Part model, mm, in its own coordinate system. Coordinates: 2 decimals unless noted, no trailing zeros. Write each loop counter-clockwise with the first axis right and the second up, starting at its lowest first coordinate (ties: lowest second). Pieces come first, ordered by that corner, then holes. Notation, with made-up numbers: (88, -9.75) -> (144, -9.75) arc R24 ccw to (144, 12.25) -> close; hole circle Ø2 at (-25.75, 19.25). An arc over 180 degrees is marked (long way). One line per question, with ' | ' between items. Start each with the question number.
Item 1: Saw through at A-A (y = 35). List the corners of the cut face in (x, z), and give its area (3 significant figures).
Item 2: Saw through at B-B (x = 141). List the corners of the cut face in (y, z), and give its area (3 significant figures).
Item 3: Probe probe 1 along Y at (x, z) = (23, 3.3); probe 2 along X at (y, z) = (54, 3); probe 3 along Y at (x, z) = (101, 1.9). List the from-to ranges inside material, lowest first. Write a range as [from, to].
Item 4: Pin check, flat tips, straight feed: pin 1 (0.9 mm diameter, centred on y = 111.5, z = 2.5, fed in from +X); pin 2 (1.5 mm diameter, centred on y = 4.5, z = 2, fed in from +X). Stop position of each tip, or through.
Item 5: Saw through at C-C (z = 0.9). List the corners of the cut face in (x, y).
from build123d import *

# Parameters (mm, degrees)
F0_W     = 162
F0_H     = 115
F0_W_2   = 151.84
F0_H_2   = 109.92
F1_DEPTH = 4
F2_R     = 6
F3_SIZE  = 12.7
F4_W     = 15
F4_H     = 4
F5_DEPTH = 6
F6_W     = 15
F6_H     = 4
F7_DEPTH = 6
F8_R     = 3


with BuildPart() as f1:
    # F0 (on Top) → F1 (new body)
    with BuildSketch(Plane.XY):
        with Locations((81, 57.5)):
            Rectangle(F0_W, F0_H)
        with Locations((81, 57.5)):
            Rectangle(F0_W_2, F0_H_2, mode=Mode.SUBTRACT)
    extrude(amount=F1_DEPTH)

    # F2
    f2_edges = [f1.edges().sort_by_distance(p)[0] for p in [
        (0, 115, 2),
        (162, 115, 2),
        (162, 0, 2),
        (0, 0, 2),
    ]]
    fillet(f2_edges, radius=F2_R)

    # F3
    f3_edges = [f1.edges().sort_by_distance(p)[0] for p in [
        (5.08, 112.46, 2),
        (156.92, 2.54, 2),
        (156.92, 112.46, 2),
        (5.08, 2.54, 2),
    ]]
    chamfer(f3_edges, length=F3_SIZE)

    # F4 (on face) → F5 (join)
    with BuildSketch(Plane(origin=(0, 2.54, 0), x_dir=(-1, 0, 0), z_dir=(0, 1, 0))):
        with Locations((-61, 2)):
            Rectangle(F4_W, F4_H)
    extrude(amount=F5_DEPTH)

    # F6 (on face) → F7 (join)
    with BuildSketch(Plane.XZ.offset(-112.46)):
        with Locations((101, 2)):
            Rectangle(F6_W, F6_H)
    extrude(amount=F7_DEPTH)

    # F8
    f8_edges = [f1.edges().sort_by_distance(p)[0] for p in [
        (93.5, 106.46, 2),
        (108.5, 106.46, 2),
        (68.5, 8.54, 2),
        (53.5, 8.54, 2),
    ]]
    fillet(f8_edges, radius=F8_R)


solid = f1.part
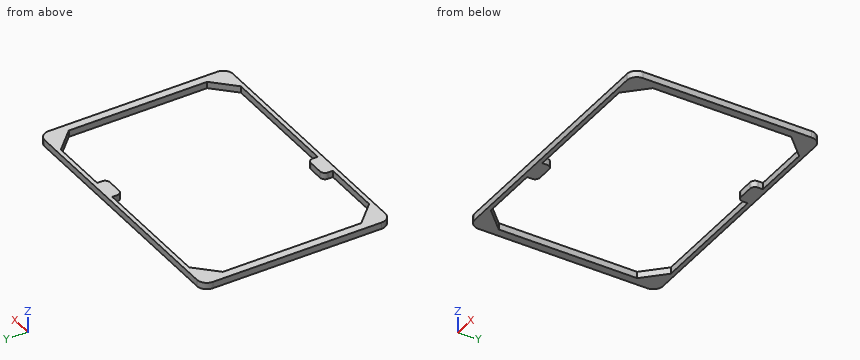
From the geometry:
1) outline: (0, 0) -> (5.08, 0) -> (5.08, 4) -> (0, 4) -> close; (156.92, 0) -> (162, 0) -> (162, 4) -> (156.92, 4) -> close | area: 40.6 mm2
2) outline: (0, 0) -> (2.54, 0) -> (2.54, 4) -> (0, 4) -> close; (112.46, 0) -> (115, 0) -> (115, 4) -> (112.46, 4) -> close | area: 20.3 mm2
3) probe 1: [0, 2.54], [112.46, 115] | probe 2: [0, 5.08], [156.92, 162] | probe 3: [0, 2.54], [106.46, 115]
4) pin 1: x = 161.64 | pin 2: x = 161.95
5) outline: (0, 6) arc R6 ccw to (6, 0) -> (156, 0) arc R6 ccw to (162, 6) -> (162, 109) arc R6 ccw to (156, 115) -> (6, 115) arc R6 ccw to (0, 109) -> close; hole (5.08, 15.24) -> (17.78, 2.54) -> (53.5, 2.54) -> (53.5, 5.54) arc R3 cw to (56.5, 8.54) -> (65.5, 8.54) arc R3 cw to (68.5, 5.54) -> (68.5, 2.54) -> (144.22, 2.54) -> (156.92, 15.24) -> (156.92, 99.76) -> (144.22, 112.46) -> (108.5, 112.46) -> (108.5, 109.46) arc R3 cw to (105.5, 106.46) -> (96.5, 106.46) arc R3 cw to (93.5, 109.46) -> (93.5, 112.46) -> (17.78, 112.46) -> (5.08, 99.76) -> close
